Autodesk Inventor part; units mm, degrees
ref_plane "YZ Plane" through (0, 0, 0) normal (1, 0, 0) x (0, 1, 0)
ref_plane "XZ Plane" through (0, 0, 0) normal (0, 1, 0) x (-1, 0, 0)
ref_plane "XY Plane" through (0, 0, 0) normal (0, 0, 1) x (1, 0, 0)
sketch "Szkic1" plane through (0, 0, 0) normal (0, 0, 1) x (1, 0, 0)
  circle A0 centre (0, 0) radius 150
  circle A1 centre (0, 0) radius 15
  circle A2 centre (0, 140) radius 4
  circle A3 centre (-70, 121.2436) radius 4
  circle A4 centre (-121.2436, 70) radius 4
  circle A5 centre (-140, 0) radius 4
  circle A6 centre (-121.2436, -70) radius 4
  circle A7 centre (-70, -121.2436) radius 4
  circle A8 centre (0, 0) radius 31
  circle A9 centre (0, -140) radius 4
  circle A10 centre (70, -121.2436) radius 4
  circle A11 centre (0, 0) radius 14
  circle A12 centre (0, 0) radius 12.5
  circle A13 centre (121.2436, -70) radius 4
  circle A14 centre (140, 0) radius 4
  circle A15 centre (121.2436, 70) radius 4
  circle A16 centre (70, 121.2436) radius 4
  circle A17 centre (0, 0) radius 92.5
  circle A18 centre (0, 0) radius 77.5
  dimension "d0" = 300
  dimension "d1" = 30
  dimension "d2" = 8
  dimension "d5" = 360
  dimension "d7" = 62
  dimension "d15" = 28
  dimension "d16" = 25
  dimension "d55" = 185
  dimension "d56" = 155
extrude "Wyciągnięcie proste1" add sketch "Szkic1" along normal blind 80 contours A1 | A11 | A12
extrude "Wyciągnięcie proste2" add sketch "Szkic1" along normal blind 12 contours A8
ref_plane "Płaszczyzna konstrukcyjna1" through (0, 0, 80) normal (0, 0, 1) x (1, 0, 0)
sketch "Szkic2" plane through (0, 0, 80) normal (0, 0, 1) x (1, 0, 0)
  circle A0 centre (0, 0) radius 8
  dimension "d21" = 16
extrude "Wyciągnięcie proste6" add sketch "Szkic2" along normal blind 25
extrude "Wyciągnięcie proste8" add sketch "Szkic1" along normal blind 10 contours A0 | A18
chamfer "Faza2" distance 1 angle 45 1 edges at (-15, 0, 80)
thread "Gwint2"
chamfer "Faza4" distance 1 angle 45 1 edges at (-8, 0, 105)
extrude "Wyciągnięcie proste9" add sketch "Szkic1" along normal blind 11.5 contours A17
sketch "Szkic10" plane through (0, 0, 0) normal (0, 0, -1) x (-1, 0, 0)
  point P0 (-1.558, -83.5832)
hole "Otwór8" at (1.558, -83.5832, 0) direction (0, 0, 1) diameter 6.6 end through all
sketch "Szkic11" plane through (0, 0, 0) normal (0, 0, -1) x (-1, 0, 0)
  point P0 (-60.2039, -58.0006)
hole "Otwór9" at (60.2039, -58.0006, 0) direction (0, 0, 1) diameter 6.6 end through all
sketch "Szkic12" plane through (0, 0, 0) normal (0, 0, -1) x (-1, 0, 0)
  point P0 (-83.5832, 1.558)
hole "Otwór10" at (83.5832, 1.558, 0) direction (0, 0, 1) diameter 6.6 end through all
sketch "Szkic13" plane through (0, 0, 0) normal (0, 0, -1) x (-1, 0, 0)
  point P0 (-58.0006, 60.2039)
hole "Otwór11" at (58.0006, 60.2039, 0) direction (0, 0, 1) diameter 6.6 end through all
sketch "Szkic14" plane through (0, 0, 0) normal (0, 0, -1) x (-1, 0, 0)
  point P0 (1.558, 83.5832)
hole "Otwór12" at (-1.558, 83.5832, 0) direction (0, 0, 1) diameter 6.6 end through all
sketch "Szkic15" plane through (0, 0, 0) normal (0, 0, -1) x (-1, 0, 0)
  point P0 (60.2039, 58.0006)
hole "Otwór13" at (-60.2039, 58.0006, 0) direction (0, 0, 1) diameter 6.6 end through all
sketch "Szkic16" plane through (0, 0, 0) normal (0, 0, -1) x (-1, 0, 0)
  point P0 (83.5832, -1.558)
hole "Otwór14" at (-83.5832, -1.558, 0) direction (0, 0, 1) diameter 6.6 end through all
sketch "Szkic17" plane through (0, 0, 0) normal (0, 0, -1) x (-1, 0, 0)
  point P0 (58.0006, -60.2039)
hole "Otwór15" at (-58.0006, -60.2039, 0) direction (0, 0, 1) diameter 6.6 end through all
properties part number "podstawa_Drukowanie 3D"
Check sheet for the modelled part. Datum: model origin and axes. Units: mm. A direction names the side the tool comes from. Round coordinates to 2 decimals unless told otherwise and drop trailing zeros. Order: outer loops, then holes, each group sorted by start corner. A loop starts at its lowest first (then second) coordinate and runs counter-clockwise, first axis right, second up. Notation, with made-up numbers: (-22.5, 76) -> (-0.5, 76) arc R23 ccw to (-0.5, 94) -> close; hole circle Ø11 at (87.25, -29.75). An arc over 180 degrees is marked (long way). One line per item, written item: value. Start each with the question number.
Q1. Thickness scan on line 1 (Y direction, x = 0, z = 10.5); line 2 (Y direction, x = 0, z = 7.5); line 3 (Z direction, x = 82.5, y = -121). Record the ranges inside material, lowest first.
Q2. Set-up check for faces 1 (the face through (-0.521, 136.034, 4.93)), 2 (the face through (13.3, 7.3, 12)): record each of +Z, -Z, +X, -X, +Y, -Y from which the full face is reachable in a straight line by a thin tool's end or side.
Q3. Cross-section at A-A (x = -70). Record the boundary of the cut face in (y, z) (3 decimals).
Q4. Cross-section at B-B (y = -140). Record the boundary of the cut face in (x, z), and give its area (3 significant figures).
Q5. Gauge pin test, flat ends, axial feed: pin 1 Ø13 at (x, y) = (0, -140) entering from +Z; pin 2 Ø8 at (x, z) = (2, 57.5) entering from -Y; pin 3 Ø10.5 at (x, y) = (1.56, -83.58) entering from +Z. Record the tip position at first contact, or that the pin passes through.
Q6. Mould release check, pull along Y, two halves, no side actions. Record for faces 3 (the face through (-19.527, -148.724, 4.93)), 4 (the face through (-2, 2, 0)), 5 (the face through (-1.703, 80.286, 5.83)): pulls with the +Y half, pulls with the -Y half, needs draft (parallel to the pull), parting line crosses it, or undercut.
Completed:
1. line 1: y = -92.5 to -86.49, -80.67 to -77.5, -31 to 31, 77.5 to 80.67, 86.49 to 92.5
1. line 2: y = -150 to -144, -136 to -86.49, -80.67 to 80.67, 86.49 to 136, 144 to 150
1. line 3: z = 0 to 10
2. face 1: +Z, -Z
2. face 2: +Z
3. outline: (-132.665, 0) -> (-125.244, 0) -> (-125.244, 10) -> (-132.665, 10) -> close; (-117.244, 0) -> (117.244, 0) -> (117.244, 10) -> (60.467, 10) -> (60.467, 11.5) -> (33.26, 11.5) -> (33.26, 10) -> (-33.26, 10) -> (-33.26, 11.5) -> (-60.467, 11.5) -> (-60.467, 10) -> (-117.244, 10) -> close; (125.244, 0) -> (132.665, 0) -> (132.665, 10) -> (125.244, 10) -> close
4. outline: (-53.85, 0) -> (-4, 0) -> (-4, 10) -> (-53.85, 10) -> close; (4, 0) -> (53.85, 0) -> (53.85, 10) -> (4, 10) -> close
4. area: 997 mm²
5. pin 1: stops at z = 10
5. pin 2: stops at y = -15
5. pin 3: stops at z = 11.5
6. face 3: parting line crosses it
6. face 4: needs draft
6. face 5: undercut
